from build123d import *

# Parameters (mm, degrees)
SKETCH1_R           = 17.5
BOSS_EXTRUDE1_DEPTH = 2
SKETCH2_R           = 10
BOSS_EXTRUDE2_DEPTH = 1
CUT_EXTRUDE1_DEPTH  = 6
SKETCH5_R           = 1
CUT_EXTRUDE2_DEPTH  = 0.01
CIRPATTERN1_COUNT   = 6
FILLET1_R           = 0.3


with BuildPart() as part:
    # Sketch1 → Boss-Extrude1 (new body)
    with BuildSketch(Plane.XY):
        Circle(SKETCH1_R)
    extrude(amount=BOSS_EXTRUDE1_DEPTH)

    # Sketch2 → Boss-Extrude2 (add)
    with BuildSketch(Plane(origin=(0, 0, 0), x_dir=(-1, 0, 0), z_dir=(0, 0, -1))):
        Circle(SKETCH2_R)
    extrude(amount=BOSS_EXTRUDE2_DEPTH)

    # Sketch4 → Cut-Extrude1 (cut)
    with BuildSketch(Plane.XY.offset(2)):
        with BuildLine():
            Line((-1.5, 13.5), (-1.5, 17.5))
            Line((-1.5, 17.5), (1.5, 17.5))
            Line((1.5, 17.5), (1.5, 13.5))
            ThreePointArc((1.5, 13.5), (0, 12), (-1.5, 13.5))
        make_face()
    cut_extrude1 = extrude(amount=-CUT_EXTRUDE1_DEPTH, mode=Mode.SUBTRACT)

    # Sketch5 → Cut-Extrude2 (cut)
    with BuildSketch(Plane.XY.offset(2)):
        Circle(SKETCH5_R)
    extrude(amount=-CUT_EXTRUDE2_DEPTH, mode=Mode.SUBTRACT)

    # CirPattern1: Cut-Extrude1 ×6 about axis
    cirpattern1_axis = Axis((0, 0, 0), (0, 0, 1))
    for i in range(1, CIRPATTERN1_COUNT):
        add(cut_extrude1.rotate(cirpattern1_axis, i * 360 / CIRPATTERN1_COUNT), mode=Mode.SUBTRACT)

    # Fillet1
    fillet1_edges = [part.edges().sort_by_distance(p)[0] for p in [
        (10, 0, -1),
    ]]
    fillet(fillet1_edges, radius=FILLET1_R)


solid = part.part
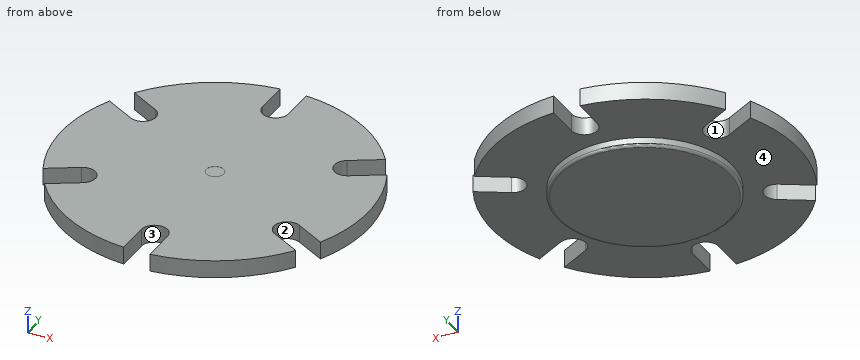
For this review, take the finished solid that the model builds, in its own axes (mm). Face numbers are marked on the shaded views. Give positions to 0.01 mm unless a question says otherwise; leave off trailing zeros. Write each loop counter-clockwise with the first axis right and the second up, starting at its lowest first coordinate (ties: lowest second). Pieces come first, ordered by that corner, then holes. Notation, with made-up numbers: (39, 23.5) -> (55, 23.5) arc R6 cw to (55, 28.5) -> close; hole circle Ø11 at (78.25, 32.25). An arc over 180 degrees is marked (long way). Use CSV: the item, a comma, the result in double quotes.
Q1. Mouldability with a two-part tool opening along Y and no side actions: class the marked faces 1, 2, 3 and 4 as pulls with the +Y half, pulls with the -Y half, needs draft (parallel to the pull), parting line crosses it, or undercut.
Conclusion:
face 1,"undercut"
face 2,"undercut"
face 3,"pulls with the -Y half"
face 4,"needs draft"
Q2. Take a section at B-B, the plane z = 0.8. Write out the cut boundary in (x, y).
Conclusion:
outline,"(-15.85, -7.42) -> (-12.44, -5.45) arc R1.5 cw to (-10.94, -8.05) -> (-14.35, -10.02) arc R17.5 ccw to (-1.5, -17.44) -> (-1.5, -13.5) arc R1.5 cw to (1.5, -13.5) -> (1.5, -17.44) arc R17.5 ccw to (14.35, -10.02) -> (10.94, -8.05) arc R1.5 cw to (12.44, -5.45) -> (15.85, -7.42) arc R17.5 ccw to (15.85, 7.42) -> (12.44, 5.45) arc R1.5 cw to (10.94, 8.05) -> (14.35, 10.02) arc R17.5 ccw to (1.5, 17.44) -> (1.5, 13.5) arc R1.5 cw to (-1.5, 13.5) -> (-1.5, 17.44) arc R17.5 ccw to (-14.35, 10.02) -> (-10.94, 8.05) arc R1.5 cw to (-12.44, 5.45) -> (-15.85, 7.42) arc R17.5 ccw to start"
Q3. To check wall thickness, follow probe 1 along Y at (x, z) = (12, 1.75); probe 2 along Z at (x, y) = (5, 16.5); probe 3 along X at (y, z) = (12.5, 0.8). State the ranges of each line that lie inside material, in increasing order. Write a range as [from, to].
Conclusion:
probe 1,"[-12.74, -8.66], [-5.28, 5.28], [8.66, 12.74]"
probe 2,"[0, 2]"
probe 3,"[-12.25, -1.12], [1.12, 12.25]"
Q4. Take a section at D-D, the plane y = -6.75. State how many separate pieces and enclosed holes the cut face has, then the cut area to 3 significant figures.
Conclusion:
separate pieces,"3"
enclosed holes,"0"
area,"61.3 mm2"
Q5. For P1, Ø0.6, axis at y = -15, z = 1, coming from the -X side; P2, Ø1.5, axis at y = -6, z = 0.5, coming from the +X side; P3, Ø1.6, axis at y = -15, z = 1.5, coming from the +X side, all flat-tipped, find the tip position at first contact; note any pin that passes through.
Conclusion:
P1,"x = -9.5"
P2,"x = 16.69"
P3,"x = 10.23"
Q6. Take a section at A-A, the plane x = 13. Write out the cut boundary in (y, z), then the cut area to 3 significant figures.
Conclusion:
outline,"(-11.72, 0) -> (-9.24, 0) -> (-9.24, 2) -> (-11.72, 2) -> close; (-5.77, 0) -> (5.77, 0) -> (5.77, 2) -> (-5.77, 2) -> close; (9.24, 0) -> (11.72, 0) -> (11.72, 2) -> (9.24, 2) -> close"
area,"33.0 mm2"
